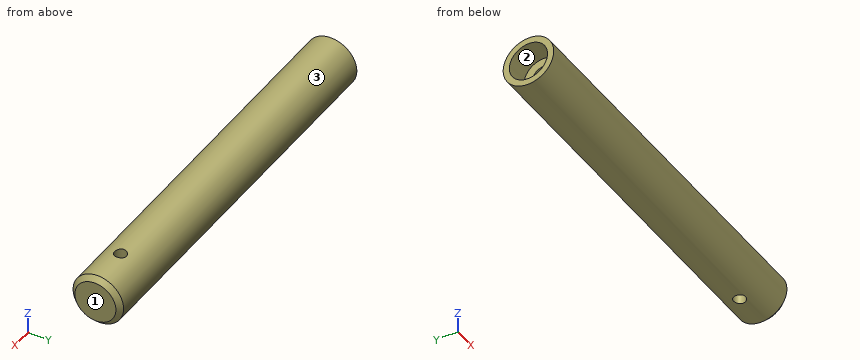
```python
from build123d import *

# Parameters (mm, degrees)
F0_R     = 2.65
F1_DEPTH = 40
F2_R     = 1.1
F3_DEPTH = 5
F4_SIZE  = 0.5
F5_R     = 0.625
F6_DEPTH = 12.5
F7_R     = 2
F8_DEPTH = 2.5


with BuildPart() as f1:
    # F0 (on Right) → F1 (new body)
    with BuildSketch(Plane.YZ):
        Circle(F0_R)
    extrude(amount=F1_DEPTH)

    # F2 (on Right) → F3 (cut)
    with BuildSketch(Plane.YZ):
        Circle(F2_R)
    extrude(amount=F3_DEPTH, mode=Mode.SUBTRACT)

    # F4
    f4_edges = [f1.edges().sort_by_distance(p)[0] for p in [
        (40, -2.65, 0),
    ]]
    chamfer(f4_edges, length=F4_SIZE)

    # F5 (on Top) → F6 (cut, symmetric)
    with BuildSketch(Plane.XY):
        with Locations((35.75, 0)):
            Circle(F5_R)
    extrude(amount=F6_DEPTH, both=True, mode=Mode.SUBTRACT)

    # F7 (on face) → F8 (cut)
    with BuildSketch(Plane(origin=(0, 0, 0), x_dir=(0, -1, 0), z_dir=(-1, 0, 0))):
        Circle(F7_R)
    extrude(amount=-F8_DEPTH, mode=Mode.SUBTRACT)


solid = f1.part
```
Read the model definition and answer for the solid it produces. Units are mm, in the model's axes. Face numbers are marked on the shaded views. Coordinates: 2 decimals unless noted, no trailing zeros. Loops run counter-clockwise (first coordinate to the right, second up) from the corner with the lowest first, then second, coordinate; pieces in that order, holes last. Notation, with made-up numbers: (53.25, 37.25) - (111.25, 37.25) arc R13 ccw to (111.25, 47.25) - close; hole circle Ø2 at (-32.5, 1). An arc over 180 degrees is marked (long way). Answer in a Markdown table with one row per item.
1. Given pin 1 (2.5 mm diameter, centred on y = 0, z = 0, fed in from -X); pin 2 (1 mm diameter, centred on x = 13, z = -1, fed in from +Y); pin 3 (0.7 mm diameter, centred on y = 0, z = 0, fed in from -X), each flat-ended and moving along its own axis, determine where each tip first touches the part or whether it passes through.
Conclusion:
| item | result |
|---|---|
| pin 1 | stops at x = 2.5 |
| pin 2 | stops at y = 2.6 |
| pin 3 | stops at x = 5 |
2. Find section A-A, the plane y = 0. Write down the section's boundary in (x, z) (3 decimals).
Conclusion:
| item | result |
|---|---|
| outline | (0, -2.65) - (35.125, -2.65) - (35.125, 2.65) - (0, 2.65) - (0, 2) - (2.5, 2) - (2.5, 1.1) - (5, 1.1) - (5, -1.1) - (2.5, -1.1) - (2.5, -2) - (0, -2) - close; (36.375, -2.65) - (39.5, -2.65) - (40, -2.15) - (40, 2.15) - (39.5, 2.65) - (36.375, 2.65) - close |
3. Determine the mould class of the marked faces 1, 2 and 3 for opening direction Z: +Z half, -Z half, draft (parallel to the pull), parting line (faces both ways), or undercut.
Conclusion:
| item | result |
|---|---|
| face 1 | draft |
| face 2 | undercut |
| face 3 | parting line |
4. Find section B-B, the plane z = 0. Write down the section's boundary in (x, y) (3 decimals).
Conclusion:
| item | result |
|---|---|
| outline | (0, -2.65) - (39.5, -2.65) - (40, -2.15) - (40, 2.15) - (39.5, 2.65) - (0, 2.65) - (0, 2) - (2.5, 2) - (2.5, 1.1) - (5, 1.1) - (5, -1.1) - (2.5, -1.1) - (2.5, -2) - (0, -2) - close; hole circle Ø1.25 at (35.75, 0) |
5. Find section C-C, the plane x = 35.75. Write down the section's boundary in (y, z) (3 decimals), then the cut area to 3 significant figures.
Conclusion:
| item | result |
|---|---|
| outline | (-0.625, -2.575) - (-0.625, 2.575) arc R2.65 ccw to start; (0.625, -2.575) arc R2.65 ccw to (0.625, 2.575) - close |
| area | 15.5 mm² |
6. Straight lines are drawn through the part: line 1 (Z direction, x = 1.65, y = 0); line 2 (Y direction, x = 35.75, z = -0.2) (3 decimals); line 3 (X direction, y = 0, z = -0.1) (3 decimals). For each, find the intervals that lie inside material, in ascending order.
Conclusion:
| item | result |
|---|---|
| line 1 | z = -2.65 to -2, 2 to 2.65 |
| line 2 | y = -2.642 to -0.625, 0.625 to 2.642 |
| line 3 | x = 5 to 35.125, 36.375 to 40 |
